from build123d import *

# Parameters (mm, degrees)
SKETCH1_W           = 89
SKETCH1_H           = 89
BOSS_EXTRUDE1_DEPTH = 8
FILLET1_R           = 3
SHELL1_T            = -2


with BuildPart() as part:
    # Sketch1 → Boss-Extrude1 (new body)
    with BuildSketch(Plane(origin=(0, 0, 0), x_dir=(1, 0, 0), z_dir=(0, 1, 0))):
        Rectangle(SKETCH1_W, SKETCH1_H)
    extrude(amount=BOSS_EXTRUDE1_DEPTH)

    # Fillet1
    fillet1_edges = [part.edges().sort_by_distance(p)[0] for p in [
        (44.5, 8, 0),
        (0, 8, -44.5),
        (-44.5, 8, 0),
        (-44.5, 4, -44.5),
        (44.5, 4, -44.5),
        (44.5, 4, 44.5),
        (-44.5, 4, 44.5),
        (0, 8, 44.5),
    ]]
    fillet(fillet1_edges, radius=FILLET1_R)

    # Shell1
    shell1_openings = [part.faces().sort_by_distance(p)[0] for p in [
        (0, 0, 0),
    ]]
    offset(amount=SHELL1_T, openings=shell1_openings, kind=Kind.INTERSECTION)


solid = part.part
Here's how the part is built. I have some questions about the finished solid (model axes, mm). A direction names the side the tool comes from. Coordinates: 2 decimals unless noted, no trailing zeros. Order: outer loops, then holes, each group sorted by start corner. A loop starts at its lowest first (then second) coordinate and runs counter-clockwise, first axis right, second up. Notation, with made-up numbers: M -0.5,77 L 56.5,77 A21 cw 56.5,108 Z; hole C 15,1 d4. An arc over 180 degrees is marked long. Answer as CSV lines item,"result". Start each with the question number.
1. I want a section at B-B, the plane z = 37.5. Write out the boundary of the cut face in (x, y), and give its area (3 significant figures).
2. I want a section at C-C, the plane x = 16.5. Write out the boundary of the cut face in (y, z), and give its area (3 significant figures).
3. We'd pull the mould along X, two halves only. Please class faces 1 (the cylindrical face through (-43.64, 2.54, -43.6)), 2 (the flat face through (-1, 6, -1)), 3 (the cylindrical face through (43.64, 7.1, -0.58)): released by +X, released by -X, zero draft, split by the parting line, or undercut.
4. On a 3-axis mill with a long thin cutter (end or side, diameter ignored), from which of +Z, -Z, +X, -X, +Y, -Y can I reach the whole of each face in a straight line? I mean faces 4 (the flat face through (42.5, 2, 1)), 5 (the cylindrical face through (0.58, 7.1, -43.64)). Say none if no direction works.
5. For pin 1 (4 mm diameter, centred on x = -27.5, z = -31, fed in from -Y), with a flat end and sliding along its axis, tell me the tip position at first contact or that it passes through.
6. I want a section at A-A, the plane y = 1.5. Write out the boundary of the cut face in (x, z).
7. I need wall thicknesses on line 1 (X direction, y = 5, z = -6); line 2 (Y direction, x = -18.5, z = 27). Which ranges of each line are inside material? Lowest first, please. Write a range as [from, to].
Recorded:
1,outline,"M -44.5,0 L -42.5,0 L -42.5,5 A1 cw -41.5,6 L 41.5,6 A1 cw 42.5,5 L 42.5,0 L 44.5,0 L 44.5,5 A3 ccw 41.5,8 L -41.5,8 A3 ccw -44.5,5 Z"
1,area,"199 mm2"
2,outline,"M 0,-44.5 L 5,-44.5 A3 ccw 8,-41.5 L 8,41.5 A3 ccw 5,44.5 L 0,44.5 L 0,42.5 L 5,42.5 A1 cw 6,41.5 L 6,-41.5 A1 cw 5,-42.5 L 0,-42.5 Z"
2,area,"199 mm2"
3,face 1,"released by -X"
3,face 2,"undercut"
3,face 3,"released by +X"
4,face 4,"-Y"
4,face 5,"-Z, +X, -X, +Y"
5,pin 1,"stops at y = 6"
6,outline,"M -44.5,-41.5 A3 ccw -41.5,-44.5 L 41.5,-44.5 A3 ccw 44.5,-41.5 L 44.5,41.5 A3 ccw 41.5,44.5 L -41.5,44.5 A3 ccw -44.5,41.5 Z; hole M -42.5,-41.5 A1 ccw -41.5,-42.5 L 41.5,-42.5 A1 ccw 42.5,-41.5 L 42.5,41.5 A1 ccw 41.5,42.5 L -41.5,42.5 A1 ccw -42.5,41.5 Z"
7,line 1,"x = [-44.5, -42.5], [42.5, 44.5]"
7,line 2,"y = [6, 8]"
